The listing builds one solid part. Answer for the finished solid, in the listing's coordinates (mm). Face numbers are marked on the shaded views. A direction names the side the tool comes from. Coordinates: 2 decimals unless noted, no trailing zeros. Order: outer loops, then holes, each group sorted by start corner. A loop starts at its lowest first (then second) coordinate and runs counter-clockwise, first axis right, second up. Notation, with made-up numbers: (11.25, 0.25) - (50.25, 0.25) arc R9 ccw to (50.25, 10.25) - close; hole circle Ø2 at (27.25, -12). An arc over 180 degrees is marked (long way). Use a Markdown table: item, result. Add a question column.
Item 1: Find the intervals of material crossed by line 1 along Y through (x, z) = (0, 1); line 2 along X through (y, z) = (7, 2.75) (3 decimals); line 3 along X through (y, z) = (-3, -3.5) (3 decimals), in increasing order.
Item 2: The part is cut by section D-D, the plane x = 0. Give the vertices of the cut face in (y, z).
Item 3: The part is cut by section B-B, the plane z = -0.75. Give the vertices of the cut face in (x, y) (3 decimals).
Item 4: The part is cut by section C-C, the plane y = -13.9. Give the vertices of the cut face in (x, z) (3 decimals), then the cut area to 3 significant figures.
Item 5: The mould has two halves that part along Z. Classify the marked faces 1, 2 and 3: released by +Z, released by -Z, zero draft, split by the parting line, or undercut.
Item 6: Flat-ended cylindrical pins translate along their axes: P1, Ø5.5, axis at x = -5, z = -10, coming from the +Y side; P2, Ø1.6, axis at x = 8.5, z = -7.5, coming from the +Y side; P3, Ø1, axis at x = 8.5, y = 2, coming from the -Z side. Find the tip coordinate at first contact, or state that the pin passes through.
Item 7: For the marked faces 4, 5 and 6, determine the directions among +Z, -Z, +X, -X, +Y, -Y from which every point of the face is accessible in a straight line to the end or side of a thin tool.
Item 8: The part is cut by section A-A, the plane x = 4.15. Give the vertices of the cut face in (y, z) (3 decimals).
Autodesk Inventor part; units mm, degrees
ref_plane "Work Plane1" through (-1.325, -11.4, 0) normal (-1, 0, 0) x (0, 0, 1)
ref_plane "Work Plane3" through (0, -16.6, 5) normal (-1, 0, 0) x (0, 0, 1)
ref_plane "YZ Plane" through (0, 0, 0) normal (1, 0, 0) x (0, 1, 0)
sketch "Sketch1" plane through (0, 0, 0) normal (0, 0, 1) x (1, 0, 0)
  line L0 (-9.975, 16.6) -> (9.975, 16.6)
  line L1 (9.975, 16.6) -> (9.975, -16.6)
  line L2 (9.975, -16.6) -> (-9.975, -16.6)
  line L3 (-9.975, -16.6) -> (-9.975, 16.6)
  line L4 (0, 0) -> (0, 11.4) construction
  line L5 (0, 0) -> (15.5803, 0) construction
  line L6 (-6.15, 11.4) -> (6.15, 11.4)
  line L7 (6.15, 11.4) -> (6.15, -11.4)
  line L8 (6.15, -11.4) -> (-6.15, -11.4)
  line L9 (-6.15, -11.4) -> (-6.15, 11.4)
  circle A0 centre (0, 13.9) radius 1.3
  circle A1 centre (0, -13.9) radius 1.3
  line L10 (-15.0861, 0) -> (20.6914, 0)
  line L11 (9.975, -16.6) -> (-9.975, -16.6)
  line L12 (-9.975, -16.6) -> (-9.975, -11.4)
  line L13 (-9.975, -11.4) -> (9.975, -11.4)
  line L14 (9.975, -11.4) -> (9.975, -16.6)
  line L15 (0, 11.4) -> (0, 13.9) construction
  point P0 (0, 16.6)
  dimension "d0" = 2.6
  dimension "d1" = 27.8
  dimension "d4" = 12.3
  dimension "d5" = 2.5
  dimension "d6" = 2.5
  dimension "d7" = 22.8
  dimension "d11" = 2.7
  dimension "d12" = 2.7
  dimension "d14" = 3.825
extrude "Extrusion1" add sketch "Sketch1" along normal blind 5 contours L0 L1 L10 L7 L6 L9 L3 | L10 L9 L13 L3 | L1 L13 L7 L10 | L13 L8 L1 L2 L3
extrude "Extrusion2" add sketch "Sketch1" against normal blind 15.8 contours L13 L8 L1 L2 L3
sketch "Sketch2" plane through (-6.15, -11.4, 5) normal (0, 1, 0) x (1, 0, 0)
  circle A0 centre (10.3, 15.485) radius 1.05
  circle A1 centre (2, 15.485) radius 1.05
  line L0 (-3.825, 20.8) -> (16.125, 20.8)
  line L1 (-3.825, 5) -> (-3.825, 20.8)
  line L2 (2, 15.485) -> (10.3, 15.485) construction
  line L3 (10.3, 15.485) -> (6.15, 15.485) construction
  line L4 (6.15, 15.485) -> (6.15, 20.8) construction
  point P0 (6.15, 5)
  dimension "d19" = 2.1
  dimension "d20" = 0
  dimension "d21" = 5.315
  dimension "d22" = 8.3
extrude "Extrusion3" cut sketch "Sketch2" against normal blind 10
sketch "Sketch3" plane through (-6.15, -11.4, 5) normal (0, 1, 0) x (1, 0, 0)
  circle A0 centre (10.3, 15.485) radius 1.05
  circle A1 centre (10.3, 15.485) radius 2.5
  circle A2 centre (2, 15.485) radius 1.05
  circle A3 centre (2, 15.485) radius 2.5
  point P0 (6.15, 5)
  dimension "d26" = 5
extrude "Extrusion4" cut sketch "Sketch3" against normal blind 2
sketch "Sketch4" plane through (9.975, -11.4, 0) normal (1, 0, 0) x (0, 0, -1)
  line L0 (0, 0) -> (15.8, 0)
  line L1 (0, 0) -> (0, 28)
  line L2 (15.8, 0) -> (0, 28)
  line L3 (0, 28) -> (0, 11.7214)
  line L4 (0, 11.7214) -> (6.6142, 0)
  line L5 (6.6142, 0) -> (15.8, 0)
  line L6 (0, 28) -> (-5, 28)
  line L7 (0, 11.7214) -> (0, 28)
  line L8 (6, 17.3671) -> (11.2857, 17.3671)
  line L9 (11.2857, 17.3671) -> (11.2857, 8)
  line L10 (11.2857, 8) -> (6, 8)
  line L11 (6, 8) -> (6, 17.3671)
  point P0 (0, 11.4)
  dimension "d29" = 8
  dimension "d33" = 8
  dimension "d34" = 6
ref_plane "Work Plane1" through (-1.325, -11.4, 0) normal (-1, 0, 0) x (0, 0, 1)
extrude "Extrusion5" add sketch "Sketch4" against normal blind 2 contours L4 L1 L2 L11 L10 L0
ref_plane "Work Plane3" through (0, -16.6, 5) normal (-1, 0, 0) x (0, 0, 1)
mirror "Mirror1" about plane through (0, -16.6, 5) normal (-1, 0, 0) of "Extrusion5"
fillet "Fillet1" radius 2 6 edges at (8.975, 0.3214, 0) (8.975, -11.4, -6.6142) (8.0625, -11.4, 0) (-8.975, -11.4, -6.6142) (-8.0625, -11.4, 0) (-8.975, 0.3214, 0)
properties part number "GrabberServoHolder_3DPrint"
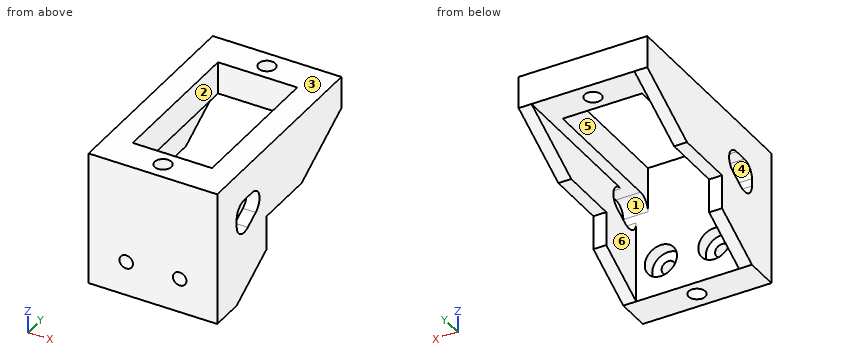
Solution:
| question | item | result |
|---|---|---|
| 1 | line 1 | y = -16.6 to -15.2, -12.6 to -11.4, 11.4 to 12.6, 15.2 to 16.6 |
| 1 | line 2 | x = -9.975 to -6.15, 6.15 to 9.975 |
| 1 | line 3 | x = -9.975 to -7.975, 7.975 to 9.975 |
| 2 | outline | (-16.6, -15.8) - (-15.2, -15.8) - (-15.2, 5) - (-16.6, 5) - close; (-12.6, -15.8) - (-11.4, -15.8) - (-11.4, 5) - (-12.6, 5) - close; (11.4, 0) - (12.6, 0) - (12.6, 5) - (11.4, 5) - close; (15.2, 0) - (16.6, 0) - (16.6, 5) - (15.2, 5) - close |
| 3 | outline | (-9.975, -16.6) - (9.975, -16.6) - (9.975, -10.961) - (6.15, -10.961) - (6.15, -11.4) - (-6.15, -11.4) - (-6.15, -10.961) - (-9.975, -10.961) - close; (-9.975, -5.731) - (-7.975, -5.731) - (-7.975, 15.271) - (-9.975, 15.271) - close; (7.975, -5.731) - (9.975, -5.731) - (9.975, 15.271) - (7.975, 15.271) - close; hole circle Ø2.6 at (0, -13.9) |
| 4 | outline | (-9.975, -15.8) - (-1.3, -15.8) - (-1.3, 5) - (-9.975, 5) - close; (1.3, -15.8) - (9.975, -15.8) - (9.975, 5) - (1.3, 5) - close; hole circle Ø2.1 at (-4.15, -10.485); hole circle Ø2.1 at (4.15, -10.485) |
| 4 | area | 354 mm2 |
| 5 | face 1 | undercut |
| 5 | face 2 | zero draft |
| 5 | face 3 | released by +Z |
| 6 | P1 | stops at y = -11.4 |
| 6 | P2 | stops at y = -3.4 |
| 6 | P3 | stops at z = -6 |
| 7 | face 4 | +X, -X |
| 7 | face 5 | +Z, -Z |
| 7 | face 6 | -Z, +Y |
| 8 | outline | (-16.6, -15.8) - (-11.4, -15.8) - (-11.4, -12.985) - (-13.4, -12.985) - (-13.4, -11.535) - (-16.6, -11.535) - close; (-16.6, -9.435) - (-13.4, -9.435) - (-13.4, -7.985) - (-11.4, -7.985) - (-11.4, 5) - (-16.6, 5) - close; (11.4, 0) - (16.6, 0) - (16.6, 5) - (11.4, 5) - close |
